from build123d import *

# Parameters (mm, degrees)
SKETCH1_R           = 2.5
BOSS_EXTRUDE1_DEPTH = 32
SKETCH1_3_R         = 2.5
BOSS_EXTRUDE2_DEPTH = 5
CUT_EXTRUDE1_START  = -32
SKETCH2_R           = 1
SKETCH2_W           = 40
SKETCH2_H           = 20
SKETCH2_R_2         = 2.5
CUT_EXTRUDE1_DEPTH  = 32
CUT_EXTRUDE2_DEPTH  = 24.2
SKETCH4_W           = 5
SKETCH4_H           = 2
CUT_EXTRUDE3_DEPTH  = 2


with BuildPart() as part:
    # Sketch1 → Boss-Extrude1 (new body)
    with BuildSketch(Plane(origin=(0, 0, 0), x_dir=(1, 0, 0), z_dir=(0, 1, 0))):
        with BuildLine():
            ThreePointArc((-35.416666667, 12.325166215), (-37.5, 0), (-35.416666667, -12.325166215))
            ThreePointArc((-35.416666667, -12.325166215), (-26.516504294, -26.516504294), (-12.325166215, -35.416666667))
            ThreePointArc((-12.325166215, -35.416666667), (0, -37.5), (12.325166215, -35.416666667))
            ThreePointArc((12.325166215, -35.416666667), (26.516504294, -26.516504294), (35.416666667, -12.325166215))
            ThreePointArc((35.416666667, -12.325166215), (36.975498644, -6.25), (37.5, 0))
            ThreePointArc((37.5, 0), (36.975498644, 6.25), (35.416666667, 12.325166215))
            ThreePointArc((35.416666667, 12.325166215), (26.516504294, 26.516504294), (12.325166215, 35.416666667))
            ThreePointArc((12.325166215, 35.416666667), (0, 37.5), (-12.325166215, 35.416666667))
            ThreePointArc((-12.325166215, 35.416666667), (-26.516504294, 26.516504294), (-35.416666667, 12.325166215))
        make_face()
        with Locations(Location((0, 0, 0), (0, 0, 270))):
            Circle(SKETCH1_R, mode=Mode.SUBTRACT)
    extrude(amount=BOSS_EXTRUDE1_DEPTH)

    # Sketch1<3> → Boss-Extrude2 (add)
    # profile 1 of 3: a face of its own
    with BuildSketch(Plane(origin=(0, 0, 0), x_dir=(1, 0, 0), z_dir=(0, 1, 0))):
        with BuildLine():
            ThreePointArc((-35.416666667, 12.325166215), (-50, 0), (-35.416666667, -12.325166215))
            ThreePointArc((-35.416666667, -12.325166215), (-37.5, 0), (-35.416666667, 12.325166215))
        make_face()
        with Locations(Location((-42.5, 0, 0), (0, 0, 270))):
            Circle(SKETCH1_3_R, mode=Mode.SUBTRACT)
    # profile 2 of 3: a face of its own
    with BuildSketch(Plane(origin=(0, 0, 0), x_dir=(1, 0, 0), z_dir=(0, 1, 0))):
        with BuildLine():
            ThreePointArc((12.325166215, -35.416666667), (0, -37.5), (-12.325166215, -35.416666667))
            ThreePointArc((-12.325166215, -35.416666667), (0, -50), (12.325166215, -35.416666667))
        make_face()
        with Locations(Location((0, -42.5, 0), (0, 0, 270))):
            Circle(SKETCH1_3_R, mode=Mode.SUBTRACT)
    # profile 3 of 3: a face of its own
    with BuildSketch(Plane(origin=(0, 0, 0), x_dir=(1, 0, 0), z_dir=(0, 1, 0))):
        with BuildLine():
            ThreePointArc((12.325166215, 35.416666667), (0, 50), (-12.325166215, 35.416666667))
            ThreePointArc((-12.325166215, 35.416666667), (0, 37.5), (12.325166215, 35.416666667))
        make_face()
        with Locations(Location((0, 42.5, 0), (0, 0, 270))):
            Circle(SKETCH1_3_R, mode=Mode.SUBTRACT)
    extrude(amount=BOSS_EXTRUDE2_DEPTH)

    # Sketch2 → Cut-Extrude1 (cut)
    # profile 1 of 5: a face of its own
    with BuildSketch(Plane(origin=(0, 32, 0), x_dir=(1, 0, 0), z_dir=(0, 1, 0)).offset(CUT_EXTRUDE1_START)):
        with Locations(Location((-35, 4.825, 0), (0, 0, 270))):
            Circle(SKETCH2_R)
    # profile 2 of 5: a face of its own
    with BuildSketch(Plane(origin=(0, 32, 0), x_dir=(1, 0, 0), z_dir=(0, 1, 0)).offset(CUT_EXTRUDE1_START)):
        with Locations(Location((-35, -4.825, 0), (0, 0, 270))):
            Circle(SKETCH2_R)
    # profile 3 of 5: a face of its own
    with BuildSketch(Plane(origin=(0, 32, 0), x_dir=(1, 0, 0), z_dir=(0, 1, 0)).offset(CUT_EXTRUDE1_START)):
        with Locations(Location((14, 4.825, 0), (0, 0, 270))):
            Circle(SKETCH2_R)
    # profile 4 of 5: a face of its own
    with BuildSketch(Plane(origin=(0, 32, 0), x_dir=(1, 0, 0), z_dir=(0, 1, 0)).offset(CUT_EXTRUDE1_START)):
        with Locations(Location((14, -4.825, 0), (0, 0, 270))):
            Circle(SKETCH2_R)
    # profile 5 of 5: a face of its own
    with BuildSketch(Plane(origin=(0, 32, 0), x_dir=(1, 0, 0), z_dir=(0, 1, 0)).offset(CUT_EXTRUDE1_START)):
        with Locations((-10.5, 0)):
            Rectangle(SKETCH2_W, SKETCH2_H)
        Circle(SKETCH2_R_2, mode=Mode.SUBTRACT)
    extrude(amount=CUT_EXTRUDE1_DEPTH, mode=Mode.SUBTRACT)

    # Sketch3 → Cut-Extrude2 (cut)
    with BuildSketch(Plane(origin=(0, 0, 0), x_dir=(-1, 0, 0), z_dir=(0, -1, 0))):
        with BuildLine():
            Line((33.018933962, -10), (38.018933962, -10))
            Line((38.018933962, -10), (38.018933962, 10))
            Line((38.018933962, 10), (33.018933962, 10))
            ThreePointArc((33.018933962, 10), (-34.5, 0), (33.018933962, -10))
        make_face()
    extrude(amount=-CUT_EXTRUDE2_DEPTH, mode=Mode.SUBTRACT)

    # Sketch4 → Cut-Extrude3 (cut)
    with BuildSketch(Plane(origin=(0, 24.2, 0), x_dir=(-1, 0, 0), z_dir=(0, -1, 0))):
        with Locations((-12, 0)):
            Rectangle(SKETCH4_W, SKETCH4_H)
        with Locations((33, 0)):
            Rectangle(SKETCH4_W, SKETCH4_H)
    extrude(amount=-CUT_EXTRUDE3_DEPTH, mode=Mode.SUBTRACT)


solid = part.part
The model under review builds one solid part; all positions refer to its coordinate system, in mm. A direction names the side the tool comes from. Round coordinates to 2 decimals unless told otherwise and drop trailing zeros. Loops run counter-clockwise (first coordinate to the right, second up) from the corner with the lowest first, then second, coordinate; pieces in that order, holes last. Notation, with made-up numbers: (-14.75, -35) -> (35.25, -35) arc R12 cw to (35.25, -16) -> close; hole circle Ø2 at (-3.5, 29.25). An arc over 180 degrees is marked (long way). Write item = value, one per line. Start each with the question number.
Item 1: Insertion check: pin 1 (1.5 mm diameter, centred on y = 13, z = 34.5, fed in from -X); pin 2 (1.6 mm diameter, centred on x = 12.5, y = 25.5, fed in from +Z); pin 3 (11.5 mm diameter, centred on x = -40.5, z = 5, fed in from +Y); pin 4 (4 mm diameter, centred on x = 16.5, y = 20.5, fed in from -Z). Each pin has a flat end and moves straight along its axis. Give the tip position at first contact, or say it passes through.
Item 2: Take a section at B-B on z = -42.5. Give the boundary of the cut face in (x, y), plus the area to 3 significant figures.
Item 3: To check wall thickness, follow L1, parallel to Z at x = -16.5, y = 31.5; L2, parallel to X at y = 4.5, z = -6.5; L3, parallel to Y at x = 4.5, z = 28. State the ranges of each line that lie inside material, in increasing order.
Item 4: Take a section at D-D on z = -8. Give the boundary of the cut face in (x, y).
Item 5: Take a section at C-C on y = 29.5. Give the boundary of the cut face in (x, z) (3 decimals).
Item 6: Mouldability with a two-part tool opening along X and no side actions: class faces 1 (the flat face through (9.5, 28, 0)), 2 (the flat face through (-30.5, 28, 0)), 3 (the cylindrical face through (0, 2, 50)), 4 (the flat face through (16, 32, -1)) as released by +X, released by -X, zero draft, split by the parting line, or undercut.
Item 7: Take a section at A-A on x = -26. Give the boundary of the cut face in (y, z).
Item 8: For faces 5 (the flat face through (-32, 0, -15)), 6 (the flat face through (-11, 28, -10)), 7 (the flat face through (-35, 12, -10)), list the 3-axis set-ups (+Z, -Z, +X, -X, +Y, -Y) from which the entire face can be reached by the end or side of a thin tool; tool diameter is ignored.
Result:
q1.pin_1 = -16.35
q1.pin_2 = 35.63
q1.pin_3 = 32
q1.pin_4 = -34.58
q2.outline = (-11.46, 0) -> (-2.5, 0) -> (-2.5, 5) -> (-11.46, 5) -> close; (2.5, 0) -> (11.46, 0) -> (11.46, 5) -> (2.5, 5) -> close
q2.area = 89.6 mm²
q3.L1 = -33.67 to -10, 10 to 33.67
q3.L2 = -48.18 to -38.02, 33.88 to 36.93
q3.L3 = 24.2 to 32
q4.outline = (-47.1, 0) -> (-38.02, 0) -> (-38.02, 5) -> (-47.1, 5) -> close; (-36.64, 24.2) -> (-30.5, 24.2) -> (-30.5, 32) -> (-36.64, 32) -> close; (9.5, 24.2) -> (33.56, 24.2) -> (33.56, 0) -> (36.64, 0) -> (36.64, 32) -> (9.5, 32) -> close
q5.outline = circle Ø75 at (0, 0); hole circle Ø2 at (-35, -4.825); hole circle Ø2 at (-35, 4.825); hole (-30.5, -10) -> (9.5, -10) -> (9.5, 10) -> (-30.5, 10) -> close; hole circle Ø2 at (14, -4.825); hole circle Ø2 at (14, 4.825)
q6.face_1 = undercut
q6.face_2 = undercut
q6.face_3 = split by the parting line
q6.face_4 = zero draft
q7.outline = (0, -27.02) -> (32, -27.02) -> (32, -10) -> (24.2, -10) -> (24.2, -22.68) -> (0, -22.68) -> close; (0, 22.68) -> (24.2, 22.68) -> (24.2, 10) -> (32, 10) -> (32, 27.02) -> (0, 27.02) -> close
q8.face_5 = +Z, -Z, +X, -X, -Y
q8.face_6 = +Y, -Y
q8.face_7 = -Y
